```python
from build123d import *

# Parameters (mm, degrees)
F0_W     = 50
F0_H     = 50
F1_DEPTH = 5
F3_DEPTH = 25


with BuildPart() as f1:
    # F0 (on Front) → F1 (new body, symmetric)
    with BuildSketch(Plane.XZ):
        Rectangle(F0_W, F0_H)
    extrude(amount=F1_DEPTH, both=True)

    # F2 (on Right) → F3 (join, symmetric)
    with BuildSketch(Plane.YZ):
        Polygon((-4.812052, -24.951309), (-4.812052, 20.26826), (-9.624103, 20.26826), (-9.624103, 14.232163), (-11.670237, 14.232163), (-11.670237, 7.070693), (-14.637132, 7.070693), (-14.637132, -4.796886), (-17.604027, -4.796886), (-17.604027, -24.951309), align=None)
    extrude(amount=F3_DEPTH, both=True)


solid = f1.part
```
The model under review builds one solid part; all positions refer to its coordinate system, in mm. A direction names the side the tool comes from. Give positions to 0.01 mm unless a question says otherwise; leave off trailing zeros. Write each loop counter-clockwise with the first axis right and the second up, starting at its lowest first coordinate (ties: lowest second). Pieces come first, ordered by that corner, then holes. Notation, with made-up numbers: M 49.5,17 L 107.5,17 A17 ccw 107.5,28 Z; hole C 33,-31 d4. An arc over 180 degrees is marked long. Write item = value, one per line. Start each with the question number.
Q1. We need section B-B (z = 17). State the section outline as (x, y) points.
Q2. Machinability: for faces 1 (the face through (0, 5, 0)), 2 (the face through (0, -11, -24.951)), 3 (the face through (0, -11, 14.232)), which of the approach directions +Z, -Z, +X, -X, +Y, -Y give a long, thin tool a straight path to every point of the face, cutting with its end or side? Answer none if there is none.
Q3. We need section C-C (z = 11.5). State the section outline as (x, y) points, plus the area to 3 significant figures.
Q4. We need section A-A (x = 11). State the section outline as (y, z) points.
Q5. For line 1 (Y direction, x = -17, z = 12); line 2 (Y direction, x = 11.5, z = 14.5); line 3 (Z direction, x = 14.5, y = -8), list the stretches that pass through material, from the lowest coordinate up.
Q6. Clearance check with flat-ended pins moving along their axes: pin 1 (2.5 mm diameter, centred on x = 1.5, y = -16.5, fed in from +Z); pin 2 (13 mm diameter, centred on x = -9, z = 2, fed in from -Y); pin 3 (2.5 mm diameter, centred on x = 1, y = -6.5, fed in from +Z). State where each tip first meets the part, or that it passes through.
Result set:
q1.outline = M -25,-9.62 L 25,-9.62 L 25,5 L -25,5 Z
q2.face_1 = +Z, -Z, +X, -X, +Y
q2.face_2 = -Z, +X, -X, -Y
q2.face_3 = +Z, +X, -X, -Y
q3.outline = M -25,-11.67 L 25,-11.67 L 25,5 L -25,5 Z
q3.area = 834 mm2
q4.outline = M -17.6,-24.95 L -5,-24.95 L -5,-25 L 5,-25 L 5,25 L -5,25 L -5,20.27 L -9.62,20.27 L -9.62,14.23 L -11.67,14.23 L -11.67,7.07 L -14.64,7.07 L -14.64,-4.8 L -17.6,-4.8 Z
q5.line_1 = -11.67 to 5
q5.line_2 = -9.62 to 5
q5.line_3 = -24.95 to 20.27
q6.pin_1 = -4.8
q6.pin_2 = -14.64
q6.pin_3 = 20.27
